Build history of the part. All positions in model axes, mm. A direction names the side the tool comes from. Round coordinates to 2 decimals unless told otherwise and drop trailing zeros. Write each loop counter-clockwise with the first axis right and the second up, starting at its lowest first coordinate (ties: lowest second). Pieces come first, ordered by that corner, then holes. Notation, with made-up numbers: (-32, 58.25) - (13, 58.25) arc R25 ccw to (13, 72.25) - close; hole circle Ø7 at (22.5, -34.5). An arc over 180 degrees is marked (long way). One line per question, with ' | ' between items.
from build123d import *

# Parameters (mm, degrees)
BOSS_EXTRUDE1_DEPTH      = 16.6624
BOSS_EXTRUDE1_DEPTH_BACK = 16.6624
CUT_EXTRUDE1_DEPTH       = 41.602962623
CUT_EXTRUDE1_DEPTH_BACK  = 41.602962623
SKETCH6_R                = 4.1656
CUT_EXTRUDE2_DEPTH       = 41.602962711


with BuildPart() as part:
    # Sketch4 → Boss-Extrude1 (new, two sides: drawn at the far end of the back side and taken through both)
    with BuildSketch(Plane.XY.offset(-BOSS_EXTRUDE1_DEPTH_BACK)):
        with BuildLine():
            Line((-19.05, 19.05), (-19.05, -19.05))
            Line((-19.05, -19.05), (19.05, -19.05))
            ThreePointArc((19.05, -19.05), (17.190128061, -14.559871939), (12.7, -12.7))
            Line((12.7, -12.7), (-4.7752, -12.7))
            ThreePointArc((-4.7752, -12.7), (-10.37887982, -10.37887982), (-12.7, -4.7752))
            Line((-12.7, -4.7752), (-12.7, 12.7))
            ThreePointArc((-12.7, 12.7), (-14.559871939, 17.190128061), (-19.05, 19.05))
        make_face()
    extrude(amount=BOSS_EXTRUDE1_DEPTH + BOSS_EXTRUDE1_DEPTH_BACK)

    # Sketch5 → Cut-Extrude1 (cut, two sides: drawn at the far end of the back side and taken through both)
    with BuildSketch(Plane(origin=(-12.7, 0, 0), x_dir=(0, 0, -1), z_dir=(1, 0, 0)).offset(-CUT_EXTRUDE1_DEPTH_BACK)):
        with BuildLine():
            Line((4.1656, 6.35), (4.1656, -6.35))
            ThreePointArc((4.1656, -6.35), (0, -10.5156), (-4.1656, -6.35))
            Line((-4.1656, -6.35), (-4.1656, 6.35))
            ThreePointArc((-4.1656, 6.35), (0, 10.5156), (4.1656, 6.35))
        make_face()
    extrude(amount=CUT_EXTRUDE1_DEPTH + CUT_EXTRUDE1_DEPTH_BACK, mode=Mode.SUBTRACT)

    # Sketch6 → Cut-Extrude2 (cut, through all)
    with BuildSketch(Plane(origin=(0, -12.7, 0), x_dir=(1, 0, 0), z_dir=(0, 1, 0))):
        with Locations(Location((0, 0, 0), (0, 0, 180))):
            Circle(SKETCH6_R)
    extrude(amount=-CUT_EXTRUDE2_DEPTH, mode=Mode.SUBTRACT)


solid = part.part
Q1. Saw through at D-D, the plane y = -16. List the corners of the cut face in (x, z), then the cut area to 3 significant figures.
Found:
outline: (-19.05, -16.66) - (18.27, -16.66) - (18.27, 16.66) - (-19.05, 16.66) - close; hole circle Ø8.33 at (0, 0) | area: 1,190 mm^2
Q2. Pull direction Z, two halves, no side cores. Call faces 4 (the flat face through (-5, -19.05, 0)), 5 (the cylindrical face through (-15.919, 10.515, 0.092)), 6 (the flat face through (-10, -11, -16.662)), 7 (the flat face through (-16, 0, -4.166)): +Z half, -Z half, draft (parallel to the pull), parting line (faces both ways), or undercut.
Found:
face 4: draft | face 5: undercut | face 6: -Z half | face 7: undercut
Q3. Which spindle directions (+Z, -Z, +X, -X, +Y, -Y) get a long thin tool onto all of the face, cutting with end or side? Do faces 1 (the cylindrical face through (-3.973, -15.831, 1.251)), 2 (the flat face through (-16, 0, 4.166)), 3 (the flat face through (6, -12.7, 0)). Say none if no direction does.
Found:
face 1: +Y, -Y | face 2: +X, -X | face 3: +Z, -Z, +X, +Y
Q4. Saw through at A-A, the plane y = 0. List the corners of the cut face in (x, z).
Found:
outline: (-19.05, -16.66) - (-12.7, -16.66) - (-12.7, -4.17) - (-19.05, -4.17) - close; (-19.05, 4.17) - (-12.7, 4.17) - (-12.7, 16.66) - (-19.05, 16.66) - close
Q5. Drop flat-ended pins along their axis: pin 1 (12 mm diameter, centred on y = -4, z = 1, fed in from +X); pin 2 (5 mm diameter, centred on y = 2, z = -5, fed in from +X); pin 3 (12 mm diameter, centred on x = 10, y = -6, fed in from +Z); pin 4 (14 mm diameter, centred on x = 6.5, z = 4.5, fed in from +Y). Give the stop position or say it passes through.
Found:
pin 1: x = -10.84 | pin 2: x = -12.7 | pin 3: through | pin 4: y = -12.7
Q6. Saw through at C-C, the plane z = 0. List the corners of the cut face in (x, y), then the cut area to 3 significant figures.
Found:
outline: (-19.05, -19.05) - (-4.17, -19.05) - (-4.17, -12.7) - (-4.78, -12.7) arc R7.92 cw to (-10.24, -10.52) - (-19.05, -10.52) - close; (-19.05, 10.52) - (-12.7, 10.52) - (-12.7, 12.7) arc R6.35 ccw to (-19.05, 19.05) - close; (4.17, -19.05) - (19.05, -19.05) arc R6.35 ccw to (12.7, -12.7) - (4.17, -12.7) - close | area: 249 mm^2
Q7. Drill centre lines: L1, parallel to Z at x = 0, y = -15; L2, parallel to Y at x = 8, z = -0.5. Where is each one in solid material? Low to high. Write a range as from..to.
Found:
L1: -16.66..-4.17, 4.17..16.66 | L2: -19.05..-12.7
